For this review, use the dimensioned drawing (mm, ordinates from the lowest corner) and the shaded views. Coordinates: 2 decimals unless noted, no trailing zeros. Loops run counter-clockwise (first coordinate to the right, second up) from the corner with the lowest first, then second, coordinate; pieces in that order, holes last. Notation, with made-up numbers: M 41,65.5 L 48,65.5 A20 cw 48,101.5 Z; hole C 25.25,80.25 d6. An arc over 180 degrees is marked long. Use CSV: the item, a comma, the result in double quotes. Start each with the question number.
1. Add section A-A, the plane y = 3.2. Write out the cut boundary in (x, z), then the cut area to 3 significant figures.
2. Add section D-D, the plane y = 0.95. Write out the cut boundary in (x, z).
3. Draft analysis for pull direction Z (two halves, no side actions). For the marked faces 1, 2, 3 and 4, state which applies: +Z half, -Z half, draft (parallel to the pull), parting line (faces both ways), or undercut.
4. Clearance check with a flat-ended pin moving along its axis: P1, Ø1.2, axis at x = 1.5, z = 12, coming from the +Y side. State where the tip first meets the part, or that it passes through.
5. Add section B-B, the plane x = 1.15. Write out the cut boundary in (y, z).
6. Add section C-C, the plane z = 10. Write out the cut boundary in (x, y).
7. For L1, parallel to Z at x = 2.65, y = 3.45; L2, parallel to Z at x = 1.2, y = 3; L3, parallel to Y at x = 2.7, z = 9.5, list the stretches that pass through material, from the lowest coordinate up.
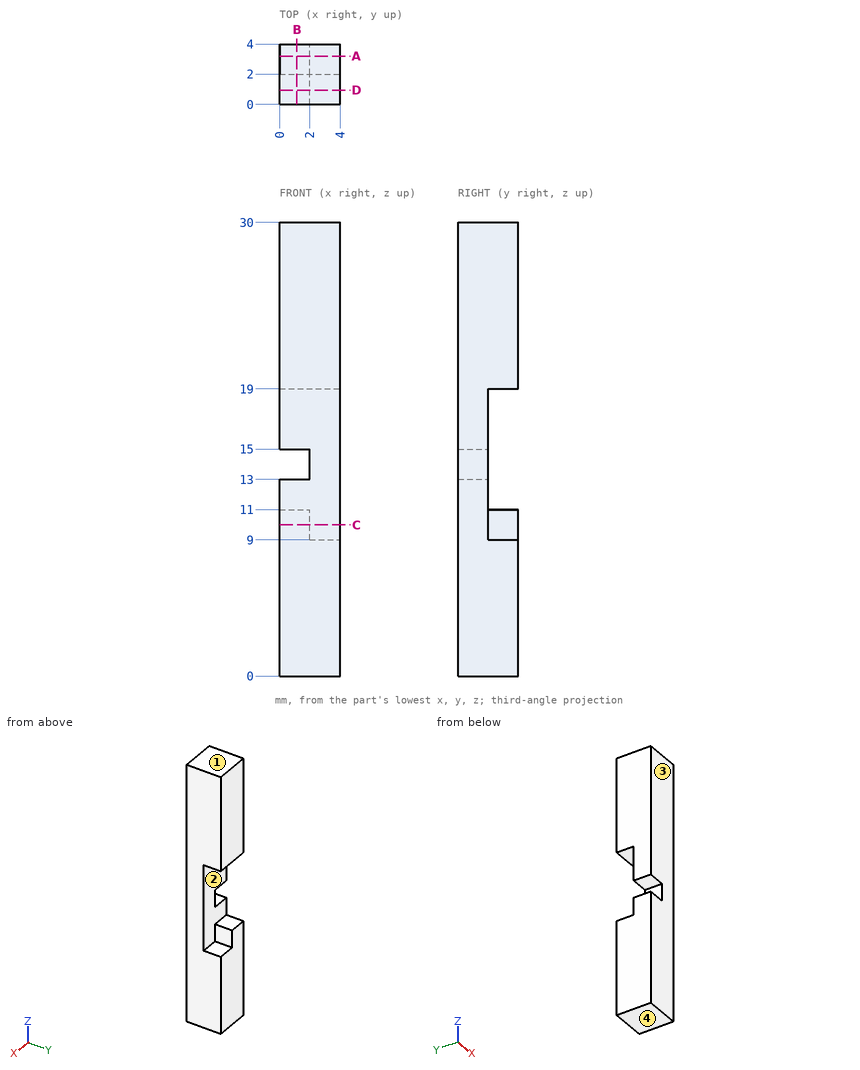
Computed:
1,outline,"M 0,0 L 4,0 L 4,9 L 2,9 L 2,11 L 0,11 Z; M 0,19 L 4,19 L 4,30 L 0,30 Z"
1,area,"84.0 mm^2"
2,outline,"M 0,0 L 4,0 L 4,30 L 0,30 L 0,15 L 2,15 L 2,13 L 0,13 Z"
3,face 1,"+Z half"
3,face 2,"undercut"
3,face 3,"draft"
3,face 4,"-Z half"
4,P1,"stops at y = 2"
5,outline,"M 0,0 L 4,0 L 4,11 L 2,11 L 2,13 L 0,13 Z; M 0,15 L 2,15 L 2,19 L 4,19 L 4,30 L 0,30 Z"
6,outline,"M 0,0 L 4,0 L 4,2 L 2,2 L 2,4 L 0,4 Z"
7,L1,"z = 0 to 9, 19 to 30"
7,L2,"z = 0 to 11, 19 to 30"
7,L3,"y = 0 to 2"
